Source: CAD feature listing. Evaluate the final solid. Frame: model axes, mm. A direction names the side the tool comes from. Round coordinates to 2 decimals unless told otherwise and drop trailing zeros. Loops run counter-clockwise (first coordinate to the right, second up) from the corner with the lowest first, then second, coordinate; pieces in that order, holes last. Notation, with made-up numbers: (10.5, 69) -> (34.5, 69) arc R28 cw to (34.5, 93) -> close; hole circle Ø2 at (39.5, -6). An arc over 180 degrees is marked (long way). Put each result on its own line as item: value. Start each with the question number.
1. Material intervals for L1, parallel to X at y = -10, z = 30.5; L2, parallel to X at y = -4.5, z = 9; L3, parallel to Z at x = -40, y = -23.5, sorted ascending.
2. Set-up query: faces 1 (the flat face through (0, -25, 25)), 2 (the flat face through (-25.4, -25, 36)). Return all of +Z, -Z, +X, -X, +Y, -Y with unobstructed straight access to the full face (end or side cutting, diameter ignored); none if empty.
3. Cut plane B-B (z = 24). Return the cut outline in (x, y), then the cut area to 3 significant figures.
4. Cut plane A-A (y = -27). Return the cut outline in (x, z), then the cut area to 3 significant figures.
5. Contact query for flat-ended pins moving along their axis: pin 1 (10 mm diameter, centred on x = -39.5, y = -9.5, fed in from +Z); pin 2 (8.5 mm diameter, centred on y = -36.5, z = 33, fed in from -X); pin 3 (3 mm diameter, centred on y = -41.5, z = 22.5, fed in from -X). Output: stop coordinate, or through.
6. Cut plane C-C (x = -38.5). Return the cut outline in (y, z).
```python
from build123d import *

# Parameters (mm, degrees)
F0_W     = 25.4
F0_H     = 50.8
F1_DEPTH = 50.8
F3_DEPTH = 50.8


with BuildPart() as f1:
    # F0 (on Front) → F1 (new body)
    with BuildSketch(Plane.XZ):
        with Locations((-12.7, 25.4)):
            Rectangle(F0_W, F0_H)
    extrude(amount=F1_DEPTH)

    # F2 (on Front) → F3 (join)
    with BuildSketch(Plane.XZ):
        Polygon((-47.622312, 0), (-22.222312, 0), (-22.222312, 25.4), align=None)
    extrude(amount=F3_DEPTH)


solid = f1.part
```
Solution:
1. L1: x = -25.4 to 0
1. L2: x = -38.62 to 0
1. L3: z = 0 to 7.62
2. face 1: +Z, -Z, +X, +Y, -Y
2. face 2: +Z, -X, +Y, -Y
3. outline: (-25.4, -50.8) -> (0, -50.8) -> (0, 0) -> (-25.4, 0) -> close
3. area: 1,290 mm^2
4. outline: (-47.62, 0) -> (0, 0) -> (0, 50.8) -> (-25.4, 50.8) -> (-25.4, 22.22) -> close
4. area: 1,540 mm^2
5. pin 1: stops at z = 13.12
5. pin 2: stops at x = -25.4
5. pin 3: stops at x = -26.62
6. outline: (-50.8, 0) -> (0, 0) -> (0, 9.12) -> (-50.8, 9.12) -> close
